Geometry: final body of the model. Coordinates: model frame, mm. Face numbers are marked on the shaded views. A direction names the side the tool comes from. Round coordinates to 2 decimals unless told otherwise and drop trailing zeros. Loops run counter-clockwise (first coordinate to the right, second up) from the corner with the lowest first, then second, coordinate; pieces in that order, holes last. Notation, with made-up numbers: M 9.25,-37 L 18.25,-37 A10 cw 18.25,-33 Z; hole C -12.75,-10 d6. An arc over 180 degrees is marked long. Return JSON: item names as keys, results as strings.
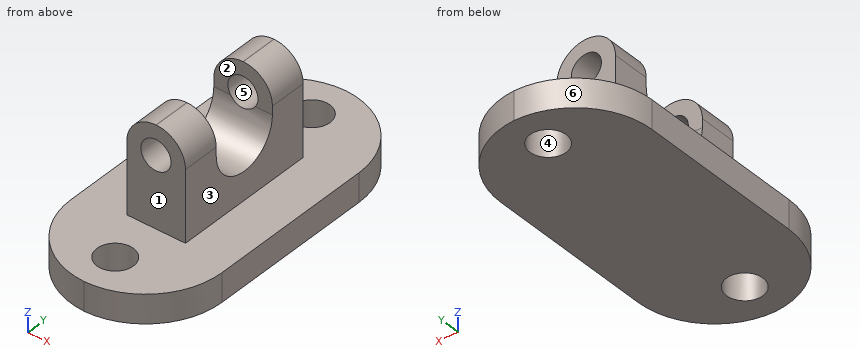
from build123d import *

# Parameters (mm, degrees)
F0_W        = 50.8
F0_H        = 108.0689131842
F1_DEPTH    = 9.652
F2_T1_DEPTH = 138.426151417
F3_R        = 6.1341
F3_R_2      = 6.1313496656
F4_DEPTH    = 9.653
F5_W        = 19.7433687763
F5_H        = 48.6069692673
F6_DEPTH    = 33.782
F7_W        = 23.2069692673
F7_H        = 12.7
F8_DEPTH    = 35.2726834568
F9_R        = 9.8113639175
F10_R       = 5.08
F11_DEPTH   = 78.3378719873


# Not quite as in the source:
# - a fillet or chamfer that OpenCascade refuses, or shapes differently, is made with other operations: its cross-section is extruded or revolved along the edge and cut away or added


with BuildPart() as f1:
    # F0 (on Top) → F1 (new body)
    with BuildSketch(Plane.XY):
        with Locations((0.4926733673, 0)):
            Rectangle(F0_W, F0_H)
    extrude(amount=F1_DEPTH)

    # F2: fillet of radius 25.7548302834 on 4 edges, made by hand

    # F2_s2 → F2_t1 (cut)
    with BuildSketch(Plane.XY.offset(-64.3870757085)):
        with BuildLine():
            ThreePointArc((25.8926733673, 28.2796263087), (18.3492582256, 46.4910414504), (0.1378430839, 54.0344565921))
            Line((0.1378430839, 54.0344565921), (25.8926733673, 54.0344565921))
            Line((25.8926733673, 54.0344565921), (25.8926733673, 28.2796263087))
        make_face()
        with BuildLine():
            ThreePointArc((0.8475036507, 54.0344565921), (-17.363911491, 46.4910414504), (-24.9073266327, 28.2796263087))
            Line((-24.9073266327, 28.2796263087), (-24.9073266327, 54.0344565921))
            Line((-24.9073266327, 54.0344565921), (0.8475036507, 54.0344565921))
        make_face()
        with BuildLine():
            ThreePointArc((0.1378430839, -54.0344565921), (18.3492582256, -46.4910414504), (25.8926733673, -28.2796263087))
            Line((25.8926733673, -28.2796263087), (25.8926733673, -54.0344565921))
            Line((25.8926733673, -54.0344565921), (0.1378430839, -54.0344565921))
        make_face()
        with BuildLine():
            ThreePointArc((0.8475036507, -54.0344565921), (-17.363911491, -46.4910414504), (-24.9073266327, -28.2796263087))
            Line((-24.9073266327, -28.2796263087), (-24.9073266327, -54.0344565921))
            Line((-24.9073266327, -54.0344565921), (0.8475036507, -54.0344565921))
        make_face()
    extrude(amount=F2_T1_DEPTH, mode=Mode.SUBTRACT)

    # F3 (on face) → F4 (cut, through all)
    with BuildSketch(Plane.XY.offset(9.652)):
        with Locations((0, -40.5962094665)):
            Circle(F3_R)
        with Locations((0, 40.5962094665)):
            Circle(F3_R_2)
    extrude(amount=-F4_DEPTH, mode=Mode.SUBTRACT)

    # F5 (on face) → F6 (join)
    with BuildSketch(Plane.XY.offset(9.652)):
        with Locations((0.4926724359, 0.0013751672)):
            Rectangle(F5_W, F5_H)
    extrude(amount=F6_DEPTH)

    # F7 (on face) → F8 (cut, through all)
    with BuildSketch(Plane.YZ.offset(10.3643568241)):
        with Locations((0.0013751672, 37.084)):
            Rectangle(F7_W, F7_H)
        with BuildLine():
            Line((11.6048598008, 30.734), (-11.6021094665, 30.734))
            ThreePointArc((-11.6021094665, 30.734), (0.0013751672, 19.1305153664), (11.6048598008, 30.734))
        make_face()
    extrude(amount=-F8_DEPTH, mode=Mode.SUBTRACT)

    # F9
    f9_edges = [f1.edges().sort_by_distance(p)[0] for p in [
        (-9.379012, 17.95486, 43.434),
        (10.364357, 17.95486, 43.434),
        (-9.379012, -17.952109, 43.434),
        (10.364357, -17.952109, 43.434),
    ]]
    fillet(f9_edges, radius=F9_R)

    # F10 (on face) → F11 (cut, through all)
    with BuildSketch(Plane(origin=(0, 24.3048598008, 0), x_dir=(-1, 0, 0), z_dir=(0, 1, 0))):
        with Locations((-0.4323519653, 33.6226360825)):
            Circle(F10_R)
    extrude(amount=-F11_DEPTH, mode=Mode.SUBTRACT)


solid = f1.part
Q1. Section query D-D (y = 4.5). Output: boundary loops of the cut face in (x, z).
Determined:
{"outline": "M -24.91,0 L 25.89,0 L 25.89,9.65 L 10.36,9.65 L 10.36,20.04 L -9.38,20.04 L -9.38,9.65 L -24.91,9.65 Z"}
Q2. Section query C-C (z = 37). Output: boundary loops of the cut face in (x, y).
Determined:
{"outline": "M -8.78,-24.3 L -3.36,-24.3 L -3.36,-11.6 L -8.78,-11.6 Z; M -8.78,11.6 L -3.36,11.6 L -3.36,24.3 L -8.78,24.3 Z; M 4.23,-24.3 L 9.76,-24.3 L 9.76,-11.6 L 4.23,-11.6 Z; M 4.23,11.6 L 9.76,11.6 L 9.76,24.3 L 4.23,24.3 Z"}
Q3. Reachability of the marked faces 1, 2 and 3 from +Z, -Z, +X, -X, +Y, -Y: full face, straight path, thin tool, end or side. Return the list, or none.
Determined:
{"face 1": "+Z, +X, -X, -Y", "face 2": "+Z, +X, -X", "face 3": "+Z, +X, +Y, -Y"}
Q4. Material intervals for L1, parallel to Y at x = 0, z = 3; L2, parallel to Y at x = -6, z = 38; L3, parallel to Z at x = -20, y = -40, sorted ascending.
Determined:
{"L1": "y = -54.02 to -46.73, -34.46 to 34.46, 46.73 to 54.02", "L2": "y = -24.3 to -11.6, 11.6 to 24.3", "L3": "z = 0 to 9.65"}
Q5. Section query A-A (x = -2). Output: boundary loops of the cut face in (y, z).
Determined:
{"outline": "M -53.88,0 L -46.4,0 L -46.4,9.65 L -53.88,9.65 Z; M -34.8,0 L 34.8,0 L 34.8,9.65 L 24.3,9.65 L 24.3,29.16 L 11.5,29.16 A11.6 cw -11.5,29.16 L -24.3,29.16 L -24.3,9.65 L -34.8,9.65 Z; M -24.3,38.08 L -11.6,38.08 L -11.6,43.13 L -24.3,43.13 Z; M 11.6,38.08 L 24.3,38.08 L 24.3,43.13 L 11.6,43.13 Z; M 46.39,0 L 53.88,0 L 53.88,9.65 L 46.39,9.65 Z"}
Q6. Section query B-B (z = 21.5). Output: boundary loops of the cut face in (x, y), plus the area to 3 significant figures.
Determined:
{"outline": "M -9.38,-24.3 L 10.36,-24.3 L 10.36,-7.03 L -9.38,-7.03 Z; M -9.38,7.03 L 10.36,7.03 L 10.36,24.3 L -9.38,24.3 Z", "area": "682 mm^2"}
Q7. Pull-direction query (Y, two-part tool) for the marked faces 4, 5 and 6; classes: pulls with the +Y half, pulls with the -Y half, needs draft (parallel to the pull), parting line crosses it, or undercut.
Determined:
{"face 4": "undercut", "face 5": "needs draft", "face 6": "pulls with the +Y half"}
Q8. Pin query (flat end, axial travel): pin 1 (8 mm diameter, centred on x = 6.5, y = 39.5, fed in from +Z); pin 2 (14 mm diameter, centred on x = -3.5, z = 35.5, fed in from +Y); pin 3 (10 mm diameter, centred on x = -2, z = 30.5, fed in from -Y). Return the tip coordinate at first contact, or that it passes through.
Determined:
{"pin 1": "stops at z = 9.65", "pin 2": "stops at y = 24.3", "pin 3": "stops at y = -24.3"}
